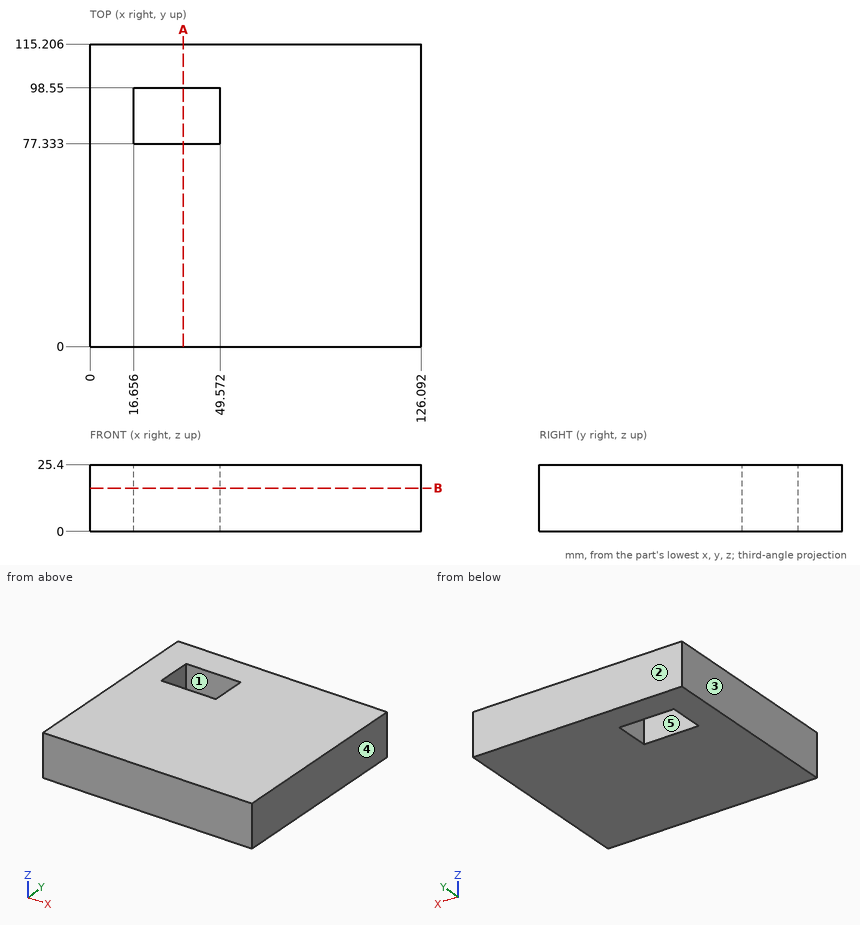
For this review, use the dimensioned drawing (mm, ordinates from the lowest corner) and the shaded views. A direction names the side the tool comes from. Coordinates: 2 decimals unless noted, no trailing zeros. Loops run counter-clockwise (first coordinate to the right, second up) from the corner with the lowest first, then second, coordinate; pieces in that order, holes last. Notation, with made-up numbers: (14, 62.5) -> (37, 62.5) arc R28 ccw to (37, 84.5) -> close; hole circle Ø2 at (78.5, 7). An arc over 180 degrees is marked (long way). Return JSON: item names as keys, results as strings. Group by question number.
(1) Consider section A-A, the plane x = 35.5. Give the boundary of the cut face in (y, z).
(2) Tool access review of the marked faces 1 and 2: name each direction out of +Z, -Z, +X, -X, +Y, -Y from which nothing blocks a thin tool from reaching the whole face with its end or side.
(3) Consider section B-B, the plane z = 16.5. Give the boundary of the cut face in (x, y), plus the area to 3 significant figures.
(4) Mouldability with a two-part tool opening along X and no side actions: class the marked faces 3, 4 and 5 as pulls with the +X half, pulls with the -X half, needs draft (parallel to the pull), parting line crosses it, or undercut.
(5) To check wall thickness, follow L1, parallel to Y at x = 49, z = 20.5; L2, parallel to X at y = 92, z = 15.5. State the ranges of each line that lie inside material, in increasing order.
Results below:
{
 "1": {"outline": "(0, 0) -> (77.33, 0) -> (77.33, 25.4) -> (0, 25.4) -> close; (98.55, 0) -> (115.21, 0) -> (115.21, 25.4) -> (98.55, 25.4) -> close"},
 "2": {"face 1": "+Z, -Z", "face 2": "+Z, -Z, +X, -X, +Y"},
 "3": {"outline": "(0, 0) -> (126.09, 0) -> (126.09, 115.21) -> (0, 115.21) -> close; hole (16.66, 77.33) -> (49.57, 77.33) -> (49.57, 98.55) -> (16.66, 98.55) -> close", "area": "13,800 mm2"},
 "4": {"face 3": "pulls with the -X half", "face 4": "pulls with the +X half", "face 5": "undercut"},
 "5": {"L1": "y = 0 to 77.33, 98.55 to 115.21", "L2": "x = 0 to 16.66, 49.57 to 126.09"}
}
